```python
from build123d import *

# Parameters (mm, degrees)
ESQUISSE1_W        = 50
ESQUISSE1_H        = 10
BOSS_EXTRU_1_DEPTH = 5


with BuildPart() as part:
    # Esquisse1 → Boss.-Extru.1 (new body)
    with BuildSketch(Plane(origin=(0, 0, 0), x_dir=(1, 0, 0), z_dir=(0, 1, 0))):
        Polygon((-25, -75), (-25, -5), (-25, 5), (-25, 25), (-35, 25), (-35, -75), align=None)
        Rectangle(ESQUISSE1_W, ESQUISSE1_H)
        Polygon((25, 5), (25, -5), (25, -75), (35, -75), (35, 25), (25, 25), align=None)
    extrude(amount=BOSS_EXTRU_1_DEPTH)


solid = part.part
```
For this review, take the finished solid that the model builds, in its own axes (mm). A direction names the side the tool comes from. Give positions to 0.01 mm unless a question says otherwise; leave off trailing zeros. Write each loop counter-clockwise with the first axis right and the second up, starting at its lowest first coordinate (ties: lowest second). Pieces come first, ordered by that corner, then holes. Notation, with made-up numbers: M 47,33 L 76,33 A20 cw 76,46 Z; hole C -38,39 d7. An arc over 180 degrees is marked long. One line per item, written item: value.
1) Take a section at A-A, the plane z = -7. Write out the cut boundary in (x, y), then the cut area to 3 significant figures.
Results are:
outline: M -35,0 L -25,0 L -25,5 L -35,5 Z; M 25,0 L 35,0 L 35,5 L 25,5 Z
area: 100 mm²
2) For faces 1 (the flat face through (-25, 2, -15)), 2 (the flat face through (-35, 2, 24)), 3 (the flat face through (-25, 2, 40)), list the 3-axis set-ups (+Z, -Z, +X, -X, +Y, -Y) from which the entire face can be reached by the end or side of a thin tool; tool diameter is ignored.
Results are:
face 1: -Z, +Y, -Y
face 2: +Z, -Z, -X, +Y, -Y
face 3: +Z, +Y, -Y
3) Take a section at C-C, the plane x = -12.5. Write out the cut boundary in (y, z), then the cut area to 3 significant figures.
Results are:
outline: M 0,-5 L 5,-5 L 5,5 L 0,5 Z
area: 50.0 mm²
4) Take a section at B-B, the plane y = 2.8. Write out the cut boundary in (x, z).
Results are:
outline: M -35,-25 L -25,-25 L -25,-5 L 25,-5 L 25,-25 L 35,-25 L 35,75 L 25,75 L 25,5 L -25,5 L -25,75 L -35,75 Z
5) The part is to be moulded in two halves that separate along X. For faces 4 (the flat face through (30, 2, 75)), 5 (the flat face through (35, 2, 26)), 6 (the flat face through (25, 2, 40)), say which applies: +X half, -X half, draft (parallel to the pull), parting line (faces both ways), or undercut.
Results are:
face 4: draft
face 5: +X half
face 6: undercut
6) For P1, Ø6, axis at x = 20.5, z = 24, coming from the +Y side; P2, Ø3, axis at x = -17, y = 4, coming from the +Z side; P3, Ø1.5, axis at x = -3.5, y = 2, coming from the -Z side, all flat-tipped, find the tip position at first contact; note any pin that passes through.
Results are:
P1: passes through
P2: stops at z = 5
P3: stops at z = -5
7) For line 1 (X direction, y = 2, z = 56.5); line 2 (Z direction, x = 11, y = 1.9), list the stretches that pass through material, from the lowest coordinate up. Write a range as from..to.
Results are:
line 1: x = -35..-25, 25..35
line 2: z = -5..5
